```python
from build123d import *

# Parameters (mm, degrees)
BOSS_EXTRUDE1_DEPTH = 5
CUT_EXTRUDE1_DEPTH  = 5


with BuildPart() as part:
    # Sketch2 → Boss-Extrude1 (new body)
    with BuildSketch(Plane.XY):
        with BuildLine():
            Line((-252.87, -75.4), (-232.15, -75.4))
            Line((-232.15, -75.4), (-232.15, -71.5))
            Line((-232.15, -71.5), (-201.961827551, -71.5))
            ThreePointArc((-201.961827551, -71.5), (-155.072329793, -49.794786091), (-141.280281757, 0))
            Line((-141.280281757, 0), (-206.208901909, 0))
            Line((-206.208901909, 0), (-252.87, -48.35711287))
            Line((-252.87, -48.35711287), (-252.87, -75.4))
        make_face()
    extrude(amount=BOSS_EXTRUDE1_DEPTH)

    # Sketch3 → Cut-Extrude1 (cut)
    with BuildSketch(Plane.XY.offset(5)):
        Polygon((-248.21, -75.4), (-244.31, -75.4), (-244.31, -71.4), (-242.86, -71.4), (-242.86, -68.4), (-244.31, -68.4), (-244.31, -62.4), (-248.21, -62.4), (-248.21, -68.4), (-249.66, -68.4), (-249.66, -71.4), (-248.21, -71.4), align=None)
        Polygon((-238.21, -75.4), (-234.31, -75.4), (-234.31, -71.4), (-232.86, -71.4), (-232.86, -68.4), (-234.31, -68.4), (-234.31, -62.4), (-238.21, -62.4), (-238.21, -68.4), (-239.66, -68.4), (-239.66, -71.4), (-238.21, -71.4), align=None)
    extrude(amount=-CUT_EXTRUDE1_DEPTH, mode=Mode.SUBTRACT)


solid = part.part
```
Build history of the part. All positions in model axes, mm. A direction names the side the tool comes from. Give positions to 0.01 mm unless a question says otherwise; leave off trailing zeros. Loops run counter-clockwise (first coordinate to the right, second up) from the corner with the lowest first, then second, coordinate; pieces in that order, holes last. Notation, with made-up numbers: (-6.75, 27) -> (21.25, 27) arc R35 cw to (21.25, 59) -> close; hole circle Ø7 at (39.25, -26). An arc over 180 degrees is marked (long way). One line per question, with ' | ' between items.
Q1. Tool access for faces 1 (the flat face through (-232.86, -70, 3)), 2 (the flat face through (-233, -75.4, 2)), 3 (the flat face through (-248.21, -73, 3)): list every direction of +Z, -Z, +X, -X, +Y, -Y with a clear straight run to the whole face (end or side of a thin tool).
Filled sheet:
face 1: +Z, -Z | face 2: +Z, -Z, +X, -X, -Y | face 3: +Z, -Z, -Y
Q2. Pull direction Y, two halves, no side cores. Call faces 4 (the flat face through (-229.21, -23.84, 2.46)), 5 (the flat face through (-242.86, -70, 3)), 6 (the flat face through (-246, -62.4, 3)), 7 (the flat face through (-239.66, -70, 3)): pulls with the +Y half, pulls with the -Y half, needs draft (parallel to the pull), parting line crosses it, or undercut.
Filled sheet:
face 4: pulls with the +Y half | face 5: undercut | face 6: pulls with the -Y half | face 7: undercut
Q3. Cut at C-C, the plane x = -229.5. Write the cut outline in (y, z).
Filled sheet:
outline: (-71.5, 0) -> (-24.14, 0) -> (-24.14, 5) -> (-71.5, 5) -> close
Q4. Drop flat-ended pins along their axis: pin 1 (3 mm diameter, centred on x = -236, z = 2, fed in from -Y); pin 2 (2 mm diameter, centred on x = -173, z = 1.5, fed in from -Y); pin 3 (2 mm diameter, centred on y = -73.5, z = 3, fed in from +X). Give the stop position or say it passes through.
Filled sheet:
pin 1: stops at y = -62.4 | pin 2: stops at y = -64.78 | pin 3: stops at x = -232.15
Q5. Cut at A-A, the plane y = -65. Write the cut outline in (x, z).
Filled sheet:
outline: (-252.87, 0) -> (-248.21, 0) -> (-248.21, 5) -> (-252.87, 5) -> close; (-244.31, 0) -> (-238.21, 0) -> (-238.21, 5) -> (-244.31, 5) -> close; (-234.31, 0) -> (-174.44, 0) -> (-174.44, 5) -> (-234.31, 5) -> close
Q6. Drill centre lines: line 1 along X through (y, z) = (-65, 2.3); line 2 along Y through (x, z) = (-203.5, 0.5); line 3 along X through (y, z) = (-63, 4.55). Where is each one in solid material? Low to high. Write a range as [from, to].
Filled sheet:
line 1: x = [-252.87, -248.21], [-244.31, -238.21], [-234.31, -174.44] | line 2: y = [-71.5, 0] | line 3: x = [-252.87, -248.21], [-244.31, -238.21], [-234.31, -170.76]
Q7. Cut at D-D, the plane y = -37.5. Write the cut outline in (x, z), plus the area to 3 significant figures.
Filled sheet:
outline: (-242.39, 0) -> (-146.95, 0) -> (-146.95, 5) -> (-242.39, 5) -> close | area: 477 mm²
